Autodesk Inventor part; units mm, degrees
ref_plane "YZ Plane" through (0, 0, 0) normal (1, 0, 0) x (0, 1, 0)
ref_plane "XZ Plane" through (0, 0, 0) normal (0, 1, 0) x (-1, 0, 0)
ref_plane "XY Plane" through (0, 0, 0) normal (0, 0, 1) x (1, 0, 0)
sketch "スケッチ1" plane through (0, 0, 0) normal (0, 0, 1) x (1, 0, 0)
  line L0 (0, 0) -> (-4, 0) construction
  circle A0 centre (-4, 0) radius 1.5
  line L1 (0, 0) -> (4, 0) construction
  circle A1 centre (4, 0) radius 1.5
  line L2 (0, 0) -> (0, 4.3) construction
  line L3 (0, 0) -> (-8.8388, 8.8388) construction
  circle A2 centre (-8.8388, 8.8388) radius 1.5
  line L4 (0, 0) -> (-8.8388, -8.8388) construction
  circle A3 centre (-8.8388, -8.8388) radius 1.5
  line L5 (0, 0) -> (8.8388, -8.8388) construction
  circle A4 centre (8.8388, -8.8388) radius 1.5
  line L6 (0, 0) -> (8.8388, 8.8388) construction
  circle A5 centre (8.8388, 8.8388) radius 1.5
  circle A6 centre (0, 0) radius 8.5
  circle A7 centre (0, 0) radius 15.5
  circle A8 centre (0, 0) radius 2
  dimension "d0" = 4
  dimension "d1" = 3
  dimension "d4" = 360
  dimension "d6" = 12.5
  dimension "d7" = 3
  dimension "d8" = 45
  dimension "d11" = 360
  dimension "d14" = 17
  dimension "d15" = 1.5
  dimension "d16" = 4
extrude "押し出し1" add sketch "スケッチ1" along normal blind 3 contours A6
sketch "スケッチ4" plane through (0, 0, 3) normal (0, 0, 1) x (1, 0, 0)
  circle A0 centre (0, 0) radius 8.5
  circle A1 centre (-4, 0) radius 1.5
  circle A2 centre (4, 0) radius 1.5
  circle A3 centre (0, 0) radius 2
  line L0 (0, 0) -> (-4.5963, 3.8567)
  line L1 (0, 0) -> (6, 0) construction
  line L2 (0, 0) -> (4.5963, 3.8567)
  line L3 (0, 0) -> (6, 0) construction
  arc A4 (4.5963, 3.8567) -> (-4.5963, 3.8567) centre (0, 0) ccw construction
  arc A5 (5.5538, 4.6602) -> (-5.5538, 4.6602) centre (0, 0) ccw
  arc A6 (3.6387, 3.0532) -> (-3.6387, 3.0532) centre (0, 0) ccw
  arc A7 (3.6387, 3.0532) -> (5.5538, 4.6602) centre (4.5963, 3.8567) ccw
  arc A8 (-5.5538, 4.6602) -> (-3.6387, 3.0532) centre (-4.5963, 3.8567) ccw
  line L4 (-4, 0) -> (4, 0)
  arc A9 (-5.5538, -4.6602) -> (5.5538, -4.6602) centre (0, 0) ccw
  arc A10 (-3.6387, -3.0532) -> (3.6387, -3.0532) centre (0, 0) ccw
  arc A11 (5.5538, -4.6602) -> (3.6387, -3.0532) centre (4.5963, -3.8567) ccw
  arc A12 (-3.6387, -3.0532) -> (-5.5538, -4.6602) centre (-4.5963, -3.8567) ccw
  dimension "d29" = 6
  dimension "d30" = 140
  dimension "d31" = 6
  dimension "d32" = 40
  dimension "d33" = 2.5
extrude "押し出し4" cut sketch "スケッチ4" against normal blind 3 contours A8 A5 A7 A6 | A12 A10 A11 A9
properties part number "脚中間フレームカム2" material "アセタール樹脂、白"
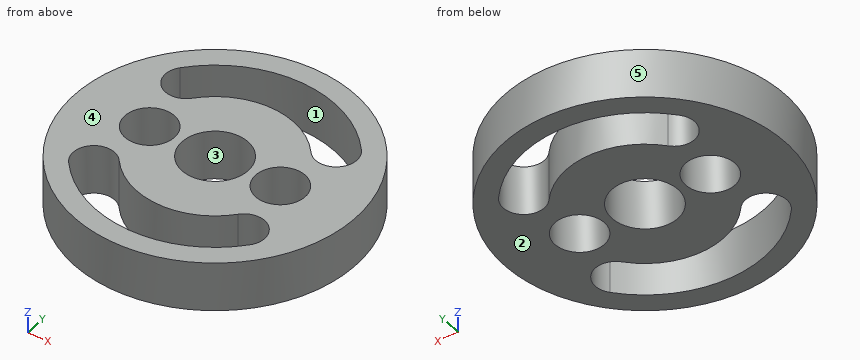
Work out the finished part from the listing and answer in its coordinate system (mm). Face numbers are marked on the shaded views. A direction names the side the tool comes from. Coordinates: 2 decimals unless noted, no trailing zeros. Loops run counter-clockwise (first coordinate to the right, second up) from the corner with the lowest first, then second, coordinate; pieces in that order, holes last. Notation, with made-up numbers: M 60,50 L 97,50 A25 cw 97,64 Z; hole C -38.5,12 d10. An arc over 180 degrees is marked long. Answer in a Markdown table with one row per item. Add a question column.
1. Find section B-B, the plane y = 6.5. Write down the section's boundary in (x, z), then the cut area to 3 significant figures.
2. Flat-ended cylindrical pins translate along their axes: P1, Ø1, axis at x = -2.5, z = 1, coming from the -Y side; P2, Ø1, axis at y = 4, z = 1.5, coming from the +X side. Find the tip coordinate at first contact, or state that the pin passes through.
3. A tool of negligible diameter and unlimited length cuts with its end or side. For the marked faces 1 and 2, from which of +Z, -Z, +X, -X, +Y, -Y can it reach the whole face along a straight path? Write none if from no direction.
4. Consider L1, parallel to Y at x = 0, z = 1.05; L2, parallel to Y at x = 4, z = 0.9; L3, parallel to X at y = 3, z = 2.1. Determine where each line is inside the solid, lowest interval first.
5. The mould has two halves that part along Y. Classify the marked faces 3, 4 and 5: pulls with the +Y half, pulls with the -Y half, needs draft (parallel to the pull), parting line crosses it, or undercut.
6. Find section A-A, the plane x = 0. Write down the section's boundary in (y, z), then the cut area to 3 significant figures.
7. Find section C-C, the plane z = 1.1. Write down the section's boundary in (x, y), then the cut area to 3 significant figures.
8. Find section D-D, the plane y = 0. Write down the section's boundary in (x, z).
Reported:
| question | item | result |
|---|---|---|
| 1 | outline | M -5.48,0 L -3.21,0 L -3.21,3 L -5.48,3 Z; M 3.21,0 L 5.48,0 L 5.48,3 L 3.21,3 Z |
| 1 | area | 13.6 mm^2 |
| 2 | P1 | stops at y = -8.26 |
| 2 | P2 | stops at x = 7.75 |
| 3 | face 1 | +Z, -Z |
| 3 | face 2 | -Z, +X, -X, +Y, -Y |
| 4 | L1 | y = -8.5 to -7.25, -4.75 to -2, 2 to 4.75, 7.25 to 8.5 |
| 4 | L2 | y = -7.5 to -6.05, -2.76 to -1.5, 1.5 to 2.76, 6.05 to 7.5 |
| 4 | L3 | x = -7.95 to -5.51, -3.69 to 3.69, 5.51 to 7.95 |
| 5 | face 3 | undercut |
| 5 | face 4 | needs draft |
| 5 | face 5 | parting line crosses it |
| 6 | outline | M -8.5,0 L -7.25,0 L -7.25,3 L -8.5,3 Z; M -4.75,0 L -2,0 L -2,3 L -4.75,3 Z; M 2,0 L 4.75,0 L 4.75,3 L 2,3 Z; M 7.25,0 L 8.5,0 L 8.5,3 L 7.25,3 Z |
| 6 | area | 24.0 mm^2 |
| 7 | outline | C 0,0 d17; hole M -5.55,-4.66 A7.25 ccw 5.55,-4.66 A1.25 ccw 3.64,-3.05 A4.75 cw -3.64,-3.05 A1.25 ccw Z; hole M -5.55,4.66 A1.25 ccw -3.64,3.05 A4.75 cw 3.64,3.05 A1.25 ccw 5.55,4.66 A7.25 ccw Z; hole C -4,0 d3; hole C 0,0 d4; hole C 4,0 d3 |
| 7 | area | 138 mm^2 |
| 8 | outline | M -8.5,0 L -5.5,0 L -5.5,3 L -8.5,3 Z; M -2.5,0 L -2,0 L -2,3 L -2.5,3 Z; M 2,0 L 2.5,0 L 2.5,3 L 2,3 Z; M 5.5,0 L 8.5,0 L 8.5,3 L 5.5,3 Z |
